from build123d import *

# Parameters (mm, degrees)
SKORUPA1_T = -0.7


with BuildPart() as part:
    # Szkic1 → Obrót1 (revolve)
    with BuildSketch(Plane.XY, mode=Mode.PRIVATE) as obr_t1_sk:
        Polygon((0, 0), (68, 0), (62, 6), (68, 12), (62, 18), (68, 24), (62, 30), (68, 36), (62, 42), (68, 48), (62, 54), (68, 60), (62, 66), (68, 72), (62, 78), (68, 84), (62, 90), (68, 96), (62, 102), (68, 108), (62, 114), (68, 120), (62, 126), (68, 132), (62, 138), (68, 144), (62, 150), (68, 156), (62, 162), (68, 168), (62, 174), (68, 180), (0, 180), align=None)
    revolve(obr_t1_sk.sketch.rotate(Axis((0, 39.738115942, 0), (0, -1, 0)), 90), axis=Axis((0, 39.738115942, 0), (0, -1, 0)))

    # Skorupa1
    skorupa1_openings = [part.faces().sort_by_distance(p)[0] for p in [
        (0, 0, 0),
        (0, 180, 0),
    ]]
    offset(amount=SKORUPA1_T, openings=skorupa1_openings, kind=Kind.INTERSECTION)


solid = part.part
Read the model definition and answer for the solid it produces. Units are mm, in the model's axes. Round coordinates to 2 decimals unless told otherwise and drop trailing zeros. Write each loop counter-clockwise with the first axis right and the second up, starting at its lowest first coordinate (ties: lowest second). Pieces come first, ordered by that corner, then holes. Notation, with made-up numbers: M -36.75,42.5 L -13.75,42.5 A17 ccw -13.75,53.5 Z; hole C 11,22 d7. An arc over 180 degrees is marked long. Use a Markdown table: item, result.
1) The part is cut by section A-A (y = 33). Write down the section's boundary in (x, z).
Answers follow:
| item | result |
|---|---|
| outline | C 0,0 d130; hole C 0,0 d128.02 |
2) Flat-ended cylindrical pins translate along their axes: pin 1 (5 mm diameter, centred on y = 132.5, z = 17, fed in from +X) (3 decimals); pin 2 (5 mm diameter, centred on y = 35, z = -10.5, fed in from -X); pin 3 (2 mm diameter, centred on y = 149.5, z = -12.5, fed in from +X). Find the tip coordinate at first contact, or state that the pin passes through.
Answers follow:
| item | result |
|---|---|
| pin 1 | stops at x = 66.425 |
| pin 2 | stops at x = -67.5 |
| pin 3 | stops at x = 62.28 |
3) Straight lines are drawn through the part: line 1 along Z through (x, y) = (39, 120.5); line 2 along X through (y, z) = (132, 15); line 3 along Z through (x, y) = (4, 21). For each, find the intervals that lie inside material, in ascending order. Write a range as [from, to].
Answers follow:
| item | result |
|---|---|
| line 1 | z = [-55.09, -53.88], [53.88, 55.09] |
| line 2 | x = [-66.32, -65.31], [65.31, 66.32] |
| line 3 | z = [-64.88, -63.88], [63.88, 64.88] |
4) For a pull along X with two mould halves and no side action, classify faces 1 (the conical face through (59.84, 113.71, -13.29)), 2 (the flat face through (45, 180, 50)), 3 (the conical face through (60.892, 30.375, -13.522)) as pulls with the +X half, pulls with the -X half, needs draft (parallel to the pull), parting line crosses it, or undercut.
Answers follow:
| item | result |
|---|---|
| face 1 | undercut |
| face 2 | needs draft |
| face 3 | parting line crosses it |
